For this review, take the finished solid that the model builds, in its own axes (mm). Round coordinates to 2 decimals unless told otherwise and drop trailing zeros. Write each loop counter-clockwise with the first axis right and the second up, starting at its lowest first coordinate (ties: lowest second). Pieces come first, ordered by that corner, then holes. Notation, with made-up numbers: M 60,53.5 L 116,53.5 A23 ccw 116,61.5 Z; hole C 64.25,85.5 d5. An arc over 180 degrees is marked long. Answer in a Markdown table with one row per item.
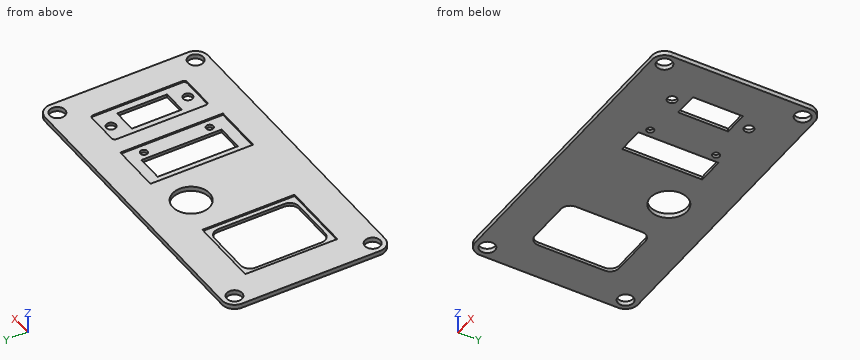
Autodesk Inventor part; units mm, degrees
ref_plane "YZ Plane" through (0, 0, 0) normal (1, 0, 0) x (0, 1, 0)
ref_plane "XZ Plane" through (0, 0, 0) normal (0, 1, 0) x (-1, 0, 0)
ref_plane "XY Plane" through (0, 0, 0) normal (0, 0, 1) x (1, 0, 0)
sketch "Sketch1" plane through (0, 0, 0) normal (0, 0, 1) x (1, 0, 0)
  line L0 (-47.5, 26.5) -> (47.5, 26.5)
  line L1 (51.5, 22.5) -> (51.5, -22.5)
  line L2 (47.5, -26.5) -> (-47.5, -26.5)
  line L3 (-51.5, -22.5) -> (-51.5, 22.5)
  arc A0 (-51.5, -22.5) -> (-47.5, -26.5) centre (-47.5, -22.5) ccw
  arc A1 (47.5, -26.5) -> (51.5, -22.5) centre (47.5, -22.5) ccw
  arc A2 (51.5, 22.5) -> (47.5, 26.5) centre (47.5, 22.5) ccw
  arc A3 (-47.5, 26.5) -> (-51.5, 22.5) centre (-47.5, 22.5) ccw
  line L4 (-47.51, 22.5) -> (47.51, 22.5) construction
  line L5 (47.51, 22.5) -> (47.51, -22.5) construction
  line L6 (47.51, -22.5) -> (-47.51, -22.5) construction
  line L7 (-47.51, -22.5) -> (-47.51, 22.5) construction
  circle A4 centre (-47.51, 22.5) radius 2.5
  circle A5 centre (47.51, 22.5) radius 2.5
  circle A6 centre (-47.51, -22.5) radius 2.5
  circle A7 centre (47.51, -22.5) radius 2.5
  point P0 (0, 0)
  point P1 (-51.5, 26.5)
  point P2 (51.5, -26.5)
  point P3 (51.5, 26.5)
  point P4 (0, 26.5)
  point P5 (51.5, 0)
  point P6 (47.51, 0)
  point P7 (0, 22.5)
  dimension "d0" = 103
  dimension "d1" = 53
  dimension "d3" = 4
  dimension "d4" = 95.02
  dimension "d5" = 45
  dimension "d6" = 5
  dimension "d7" = 5
  dimension "d8" = 5
  dimension "d9" = 5
extrude "Extrusion1" add sketch "Sketch1" along normal mid plane 1.5
sketch "Sketch2" plane through (0, 0, 0.75) normal (0, 0, 1) x (1, 0, 0)
  line L0 (47.5, 26.5) -> (-47.5, 26.5)
  point P0 (0, 0)
  point P1 (-5, 10.8)
  dimension "d51" = 5
  dimension "d52" = 15.7
hole "Neon" at (-5, 10.8, 0.75) direction (0, 0, -1) diameter 12 end through all
sketch "Sketch3" plane through (0, 0, 0.75) normal (0, 0, 1) x (1, 0, 0)
  line L0 (-36.3319, 13.6885) -> (-22.3319, 13.6885)
  line L1 (-19.3319, 10.6885) -> (-19.3319, -10.8115)
  line L2 (-22.3319, -13.8115) -> (-36.3319, -13.8115)
  line L3 (-39.3319, -10.8115) -> (-39.3319, 10.6885)
  arc A0 (-36.3319, 13.6885) -> (-39.3319, 10.6885) centre (-36.3319, 10.6885) ccw
  arc A1 (-19.3319, 10.6885) -> (-22.3319, 13.6885) centre (-22.3319, 10.6885) ccw
  arc A2 (-22.3319, -13.8115) -> (-19.3319, -10.8115) centre (-22.3319, -10.8115) ccw
  arc A3 (-39.3319, -10.8115) -> (-36.3319, -13.8115) centre (-36.3319, -10.8115) ccw
  line L4 (-40.8319, 14.9385) -> (-17.8319, 14.9385)
  line L5 (-17.8319, 14.9385) -> (-17.8319, -15.0615)
  line L6 (-17.8319, -15.0615) -> (-40.8319, -15.0615)
  line L7 (-40.8319, -15.0615) -> (-40.8319, 14.9385)
  point P0 (0, 0)
  point P1 (-39.3319, 13.6885)
  point P2 (-19.3319, -13.8115)
  point P3 (-19.3319, 13.6885)
  point P4 (-17.8319, -0.0615)
  point P5 (-19.3319, -0.0615)
  point P6 (-29.3319, 14.9385)
  point P7 (-29.3319, 13.6885)
  dimension "d20" = 20
  dimension "d21" = 27.5
  dimension "d22" = 3
  dimension "d37" = 30
  dimension "d38" = 23
extrude "IEC" cut sketch "Sketch3" against normal through all contours L0 A1 L1 A2 L2 A3 L3 A0
sketch "Sketch4" plane through (0, 0, 0.75) normal (0, 0, 1) x (1, 0, 0)
  line L0 (39.1106, 8.15) -> (31.2106, 8.15)
  line L1 (31.2106, 8.15) -> (31.2106, -8.15)
  line L2 (31.2106, -8.15) -> (39.1106, -8.15)
  line L3 (39.1106, -8.15) -> (39.1106, 8.15)
  circle A0 centre (35.1606, 12.5) radius 1.55
  circle A1 centre (35.1606, -12.5) radius 1.55
  line L4 (35.1606, 12.5) -> (35.1606, -12.5) construction
  line L5 (29.9106, 15.5) -> (40.4106, 15.5)
  line L6 (41.4106, 14.5) -> (41.4106, -14.5)
  line L7 (40.4106, -15.5) -> (29.9106, -15.5)
  line L8 (28.9106, -14.5) -> (28.9106, 14.5)
  arc A2 (41.4106, 14.5) -> (40.4106, 15.5) centre (40.4106, 14.5) ccw
  arc A3 (29.9106, 15.5) -> (28.9106, 14.5) centre (29.9106, 14.5) ccw
  arc A4 (28.9106, -14.5) -> (29.9106, -15.5) centre (29.9106, -14.5) ccw
  arc A5 (40.4106, -15.5) -> (41.4106, -14.5) centre (40.4106, -14.5) ccw
  point P0 (0, 0)
  point P1 (35.1606, 8.15)
  point P2 (35.1606, -8.15)
  point P3 (35.1606, 0)
  point P4 (39.1106, 0)
  point P5 (41.4106, 0)
  point P6 (35.1606, 15.5)
  dimension "d25" = 7.9
  dimension "d26" = 16.3
  dimension "d27" = 3.1
  dimension "d28" = 3.1
  dimension "d29" = 25
  dimension "d30" = 1
  dimension "d31" = 31
  dimension "d32" = 12.5
extrude "SUB-D" cut sketch "Sketch4" against normal through all contours L3 L2 L1 L0 | A0 | A1
extrude "Extrusion4" cut sketch "Sketch4" against normal blind 0.5
extrude "Extrusion5" cut sketch "Sketch3" against normal blind 0.5
sketch "Sketch5" plane through (0, 0, 0.75) normal (0, 0, 1) x (1, 0, 0)
  line L0 (7.0815, 16.72) -> (23.2815, 16.72)
  line L1 (23.2815, 16.72) -> (23.2815, -16.72)
  line L2 (23.2815, -16.72) -> (7.0815, -16.72)
  line L3 (7.0815, -16.72) -> (7.0815, 16.72)
  line L4 (9.2315, 13.05) -> (17.9315, 13.05)
  line L5 (17.9315, 13.05) -> (17.9315, -13.05)
  line L6 (17.9315, -13.05) -> (9.2315, -13.05)
  line L7 (9.2315, -13.05) -> (9.2315, 13.05)
  line L8 (20.4815, 10.715) -> (20.4815, -10.715) construction
  circle A0 centre (20.4815, 10.715) radius 1.15
  circle A1 centre (20.4815, -10.715) radius 1.15
  point P0 (0, 0)
  point P1 (17.9315, 0)
  point P2 (23.2815, 0)
  point P3 (20.4815, 0)
  point P4 (7.0815, 0)
  dimension "d41" = 16.2
  dimension "d42" = 33.44
  dimension "d43" = 8.7
  dimension "d44" = 14.05
  dimension "d45" = 2.8
  dimension "d46" = 21.43
  dimension "d47" = 26.1
  dimension "d48" = 2.3
  dimension "d49" = 2.3
extrude "Extrusion6" cut sketch "Sketch5" against normal through all contours L4 L5 L6 L7 | A0 | A1
extrude "Extrusion7" cut sketch "Sketch5" against normal blind 0.5
properties part number "Paneeltje"
Q1. Take a section at D-D (x = -5). State the section outline as (y, z) points, then the cut area to 3 significant figures.
Found:
| item | result |
|---|---|
| outline | M -26.5,-0.75 L 4.8,-0.75 L 4.8,0.75 L -26.5,0.75 Z; M 16.8,-0.75 L 26.5,-0.75 L 26.5,0.75 L 16.8,0.75 Z |
| area | 61.5 mm² |
Q2. Take a section at B-B (y = -0.5). State the section outline as (x, z) points.
Found:
| item | result |
|---|---|
| outline | M -51.5,-0.75 L -39.33,-0.75 L -39.33,0.25 L -40.83,0.25 L -40.83,0.75 L -51.5,0.75 Z; M -19.33,-0.75 L 9.23,-0.75 L 9.23,0.25 L 7.08,0.25 L 7.08,0.75 L -17.83,0.75 L -17.83,0.25 L -19.33,0.25 Z; M 17.93,-0.75 L 31.21,-0.75 L 31.21,0.25 L 28.91,0.25 L 28.91,0.75 L 23.28,0.75 L 23.28,0.25 L 17.93,0.25 Z; M 39.11,-0.75 L 51.5,-0.75 L 51.5,0.75 L 41.41,0.75 L 41.41,0.25 L 39.11,0.25 Z |
Q3. For probe 1 along X at (y, z) = (-11, 0.3); probe 2 along Y at (x, z) = (-47.51, -0.25); probe 3 along X at (y, z) = (2, -0.05), list the stretches that pass through material, from the lowest coordinate up.
Found:
| item | result |
|---|---|
| probe 1 | -51.5 to -40.83, -17.83 to 7.08, 23.28 to 28.91, 41.41 to 51.5 |
| probe 2 | -26.5 to -25, -20 to 20, 25 to 26.5 |
| probe 3 | -51.5 to -39.33, -19.33 to 9.23, 17.93 to 31.21, 39.11 to 51.5 |
Q4. Take a section at A-A (x = -34.5). State the section outline as (y, z) points.
Found:
| item | result |
|---|---|
| outline | M -26.5,-0.75 L -13.81,-0.75 L -13.81,0.25 L -15.06,0.25 L -15.06,0.75 L -26.5,0.75 Z; M 13.69,-0.75 L 26.5,-0.75 L 26.5,0.75 L 14.94,0.75 L 14.94,0.25 L 13.69,0.25 Z |
Q5. Insertion check: P1, Ø6.5, axis at x = 32.5, y = 5.5, coming from the +Z side; P2, Ø1.4, axis at x = 20.48, y = -10.72, coming from the -Z side. Each pin has a flat end and moves straight along its axis. Give the tip position at first contact, or say it passes through.
Found:
| item | result |
|---|---|
| P1 | z = 0.25 |
| P2 | through |
Q6. Take a section at C-C (y = -21.5). State the section outline as (x, z) points.
Found:
| item | result |
|---|---|
| outline | M -51.5,-0.75 L -49.8,-0.75 L -49.8,0.75 L -51.5,0.75 Z; M -45.22,-0.75 L 45.22,-0.75 L 45.22,0.75 L -45.22,0.75 Z; M 49.8,-0.75 L 51.5,-0.75 L 51.5,0.75 L 49.8,0.75 Z |
